```python
from build123d import *

# Parameters (mm, degrees)
F1_DEPTH = 101.6
F2_W     = 47.920428
F2_H     = 39.289536
F3_DEPTH = 13.208


with BuildPart() as f1:
    # F0 (on Right) → F1 (new body)
    with BuildSketch(Plane.YZ):
        Polygon((9.772886, -18.784101), (-28.327114, -18.784101), (-28.327114, -31.484101), (35.172886, -31.484101), (35.172886, 32.015899), (9.772886, 32.015899), align=None)
    extrude(amount=-F1_DEPTH)

    # F2 (on face) → F3 (cut)
    with BuildSketch(Plane.XZ.offset(-9.772886)):
        with Locations((-52.063208, 12.371131)):
            Rectangle(F2_W, F2_H)
    extrude(amount=-F3_DEPTH, mode=Mode.SUBTRACT)


solid = f1.part
```
Verification items for the finished model (mm, model axes). A direction names the side the tool comes from. Round coordinates to 2 decimals unless told otherwise and drop trailing zeros. Loops run counter-clockwise (first coordinate to the right, second up) from the corner with the lowest first, then second, coordinate; pieces in that order, holes last. Notation, with made-up numbers: (-12, 75.5) -> (29, 75.5) arc R33 ccw to (29, 111.5) -> close; hole circle Ø11 at (85.25, 48). An arc over 180 degrees is marked (long way). Answer as a JSON object with one key per item and string values.
Q1. Section check C-C (y = -16). Record the boundary of the cut face in (x, z).
Data:
{"outline": "(-101.6, -31.48) -> (0, -31.48) -> (0, -18.78) -> (-101.6, -18.78) -> close"}
Q2. Section check D-D (x = -85.5). Record the boundary of the cut face in (y, z).
Data:
{"outline": "(-28.33, -31.48) -> (35.17, -31.48) -> (35.17, 32.02) -> (9.77, 32.02) -> (9.77, -18.78) -> (-28.33, -18.78) -> close"}
Q3. Section check A-A (x = -41). Record the boundary of the cut face in (y, z).
Data:
{"outline": "(-28.33, -31.48) -> (35.17, -31.48) -> (35.17, 32.02) -> (22.98, 32.02) -> (22.98, -7.27) -> (9.77, -7.27) -> (9.77, -18.78) -> (-28.33, -18.78) -> close"}
Q4. Go/stop test with flat-tipped pins: P1, Ø19.5, axis at x = -60.5, z = 9.5, coming from the -Y side; P2, Ø1.5, axis at x = -89, y = 6, coming from the +Z side; P3, Ø1, axis at x = -90, z = -9.5, coming from the -Y side; P4, Ø10, axis at y = 4.5, z = -13, coming from the +X side. Record where each tip stops, or that it passes through.
Data:
{"P1": "stops at y = 22.98", "P2": "stops at z = -18.78", "P3": "stops at y = 9.77", "P4": "passes through"}
Q5. Section check B-B (z = 18.5). Record the boundary of the cut face in (x, y).
Data:
{"outline": "(-101.6, 9.77) -> (-76.02, 9.77) -> (-76.02, 22.98) -> (-28.1, 22.98) -> (-28.1, 9.77) -> (0, 9.77) -> (0, 35.17) -> (-101.6, 35.17) -> close"}
Q6. Access from +Z, -Z, +X, -X, +Y, -Y to the whole of each face (thin tool, end or side, straight path). Record for faces 1 (the flat face through (-50, 9.773, -10)), 2 (the flat face through (-28.103, 16, 12)), 3 (the flat face through (-50, 35.173, 0)).
Data:
{"face 1": "+Z, +X, -X, -Y", "face 2": "+Z, -Y", "face 3": "+Z, -Z, +X, -X, +Y"}
Q7. Scan lines: line 1 (X direction, y = 20.5, z = -4.5); line 2 (Z direction, x = -74, y = 20); line 3 (Y direction, x = -91.5, z = 1.5). Record each from-to range of solid material in increasing order. Write a range as from..to.
Data:
{"line 1": "x = -101.6..-76.02, -28.1..0", "line 2": "z = -31.48..-7.27", "line 3": "y = 9.77..35.17"}
Q8. Draft check along X on faces 4 (the flat face through (-76.023, 16, 12)), 5 (the flat face through (-52, 16, -7.274)), 6 (the flat face through (0, 17, -6)), 7 (the flat face through (-50, -28.327, -25)). Enter one of: pulls with the +X half, pulls with the -X half, needs draft (parallel to the pull), parting line crosses it, or undercut.
Data:
{"face 4": "undercut", "face 5": "undercut", "face 6": "pulls with the +X half", "face 7": "needs draft"}
